Design review of the part shown in the three views and the two pictorial views. Dimensions are in mm from the part's minimum x, y and z. Give positions to 0.01 mm unless a question says otherwise; leave off trailing zeros. Order: outer loops, then holes, each group sorted by start corner. A loop starts at its lowest first (then second) coordinate and runs counter-clockwise, first axis right, second up. Notation, with made-up numbers: M -31.75,45.5 L 7.25,45.5 A12 cw 7.25,55.5 Z; hole C 56,11.5 d5. An arc over 180 degrees is marked long. Answer as a JSON object with one key per item and string values.
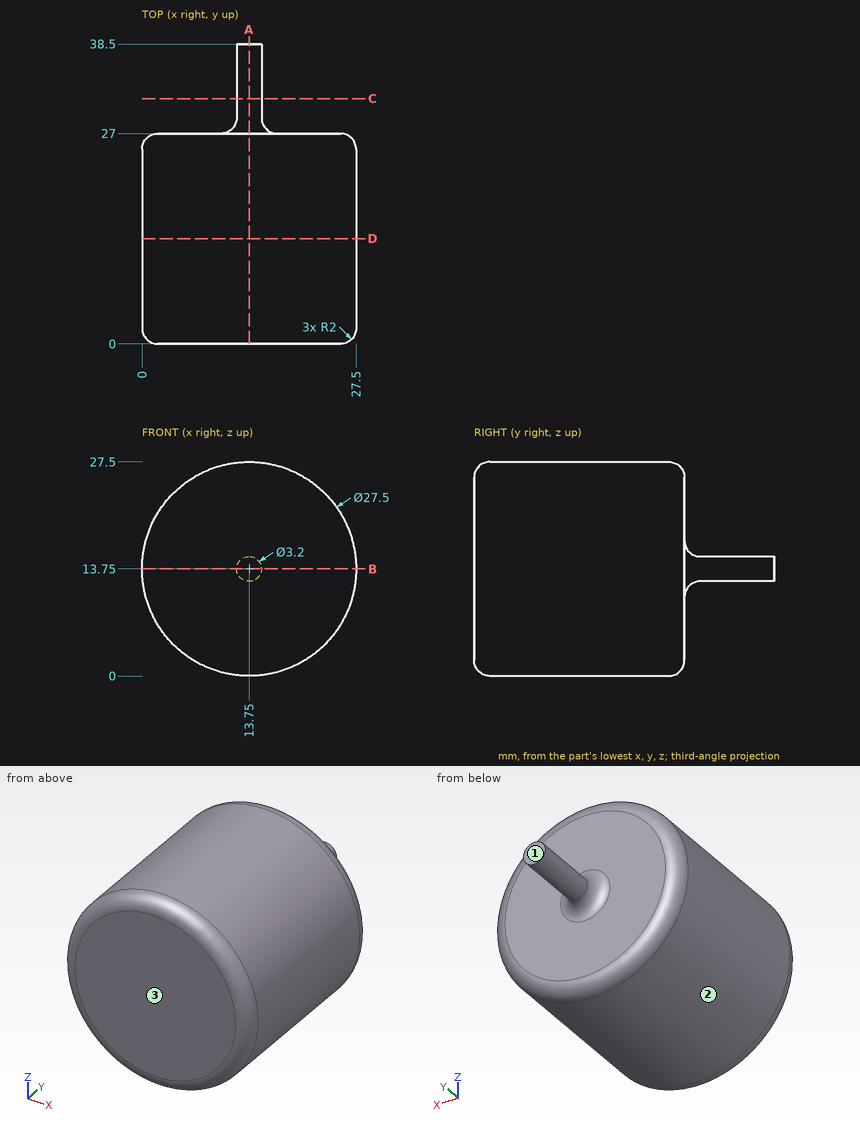
(1) We need section D-D (y = 13.5). Write out the cut boundary in (x, z), plus the area to 3 significant figures.
Checked values:
{"outline": "C 13.75,13.75 d27.5", "area": "594 mm^2"}
(2) We need section B-B (z = 13.75). Write out the cut boundary in (x, y), plus the area to 3 significant figures.
Checked values:
{"outline": "M 0,2 A2 ccw 2,0 L 25.5,0 A2 ccw 27.5,2 L 27.5,25 A2 ccw 25.5,27 L 17.35,27 A2 cw 15.35,29 L 15.35,38.5 L 12.15,38.5 L 12.15,29 A2 cw 10.15,27 L 2,27 A2 ccw 0,25 Z", "area": "778 mm^2"}
(3) To check wall thickness, follow L1, parallel to Y at x = 3.25, z = 10.5; L2, parallel to X at y = 17, z = 3.5; L3, parallel to Z at x = 26.25, y = 20. State the ranges of each line that lie inside material, in increasing order. Write a range as from..to.
Checked values:
{"L1": "y = 0..27", "L2": "x = 4.58..22.92", "L3": "z = 8.02..19.48"}
(4) Insertion check: pin 1 (1 mm diameter, centred on x = 22.5, y = 5.5, fed in from +Z); pin 2 (7 mm diameter, centred on x = 18.5, z = 19.5, fed in from +Y); pin 3 (3 mm diameter, centred on y = 9.5, z = 10, fed in from -X); pin 4 (8 mm diameter, centred on x = 22, y = 32, fed in from -Z). Each pin has a flat end and moves straight along its axis. Give the tip position at first contact, or say it passes through.
Checked values:
{"pin 1": "stops at z = 24.75", "pin 2": "stops at y = 27", "pin 3": "stops at x = 0.19", "pin 4": "passes through"}
(5) We need section C-C (y = 31.5). Write out the cut boundary in (x, z).
Checked values:
{"outline": "C 13.75,13.75 d3.2"}
(6) We need section A-A (x = 13.75). Write out the cut boundary in (y, z), plus the area to 3 significant figures.
Checked values:
{"outline": "M 0,2 A2 ccw 2,0 L 25,0 A2 ccw 27,2 L 27,10.15 A2 cw 29,12.15 L 38.5,12.15 L 38.5,15.35 L 29,15.35 A2 cw 27,17.35 L 27,25.5 A2 ccw 25,27.5 L 2,27.5 A2 ccw 0,25.5 Z", "area": "778 mm^2"}
(7) Draft analysis for pull direction Y (two halves, no side actions). For the marked faces 1, 2 and 3, state which applies: +Y half, -Y half, draft (parallel to the pull), parting line (faces both ways), or undercut.
Checked values:
{"face 1": "+Y half", "face 2": "draft", "face 3": "-Y half"}
